Input: part model. Units: mm. Frame: model coordinates. A direction names the side the tool comes from. Coordinates: 2 decimals unless noted, no trailing zeros. Loops run counter-clockwise (first coordinate to the right, second up) from the corner with the lowest first, then second, coordinate; pieces in that order, holes last.
(1) Mould query, pull axis Y, two halves, no side actions, for faces 4 (the face through (-5.6, 9.4, -6)), 5 (the face through (2, 9, 3.175)), 6 (the face through (3, 9, 0)). Classes: released by +Y, released by -Y, zero draft, split by the parting line, or undercut.
(2) Section B-B, the plane x = 5. Return loops of the section in (y, z) (3 decimals), then the cut area to 3 significant figures.
(3) Contact query for flat-ended pins moving along their axis: P1, Ø5, axis at x = -4, z = -1.5, coming from the -Y side; P2, Ø0.6, axis at x = 3.5, y = 8.5, coming from the +Z side; P3, Ø3, axis at x = -3, y = 9, coming from the +Z side; P4, Ø3.5, axis at y = 5.7, z = -6.05, coming from the +X side. Output: stop coordinate, or through.
(4) Section A-A, the plane z = -6.05. Return loops of the section in (x, y), then the cut area to 3 significant figures.
(5) Set-up query: faces 1 (the face through (3.1, 9.5, 1.6)), 2 (the face through (3, 3, 0)), 3 (the face through (6.35, 8, -5)). Return all of +Z, -Z, +X, -X, +Y, -Y with unobstructed straight access to the full face (end or side cutting, diameter ignored); none if empty.
(6) Line query: L1, parallel to Y at x = 2.75, z = -6.05; L2, parallel to X at y = 9.5, z = -5; L3, parallel to Z at x = 1, y = 5.75 (3 decimals). Output: solid intervals per line, ascending.
(7) Section C-C, the plane y = 7.25. Return loops of the section in (x, z) (3 decimals), then the cut area to 3 significant figures.
Autodesk Inventor part; units mm, degrees
ref_plane "YZ Plane" through (0, 0, 0) normal (1, 0, 0) x (0, 1, 0)
ref_plane "XZ Plane" through (0, 0, 0) normal (0, 1, 0) x (-1, 0, 0)
ref_plane "XY Plane" through (0, 0, 0) normal (0, 0, 1) x (1, 0, 0)
sketch "Sketch1" plane through (0, 0, 0) normal (1, 0, 0) x (0, 1, 0)
  line L0 (0, 0) -> (11.4, 0)
  line L1 (11.4, 0) -> (11.4, -12.1)
  line L2 (11.4, -12.1) -> (0, -12.1)
  line L3 (0, -12.1) -> (0, 0)
  arc A0 (11.4, -2.9512) -> (11.4, -9.1488) centre (12.8006, -6.05) ccw
  point P0 (3.5, -5)
  dimension "d0" = 11.4
  dimension "d1" = 12.1
  dimension "d2" = 6.1976
  dimension "d3" = 2.9512
  dimension "d29" = 2
extrude "Extrusion1" add sketch "Sketch1" along normal blind 6.35
extrude "Extrusion2" add sketch "Sketch1" against normal blind 11.43 contours L1 A0
sketch "Sketch3" plane through (0, 0, 0) normal (-1, 0, 0) x (0, 0, 1)
  line L0 (0, 11.4) -> (0, 0)
  line L1 (0, 0) -> (-12.1, 0)
  point P0 (-6.05, 5.7)
  dimension "d19" = 12.1
  dimension "d20" = 6.05
  dimension "d30" = 11.4
  dimension "d31" = 5.7
sketch "Sketch6" plane through (0, 0, 0) normal (0, 0, 1) x (1, 0, 0)
  line L0 (6.35, 5.7) -> (0, 5.7)
  line L1 (0, 0) -> (0, 11.4)
  line L2 (6.35, 11.4) -> (6.35, 0)
  line L3 (0, 0) -> (6.35, 0)
  line L4 (0, 11.4) -> (6.35, 11.4)
  dimension "d33" = 11.4
  dimension "d46" = 5.7
hole "Hole2" at (0, 5.7, -6.05) direction (1, 0, 0) diameter 4 end through all
extrude "Extrusion8" add sketch "Sketch6" along normal blind 3.175 contours L0 L1 L4 L2
sketch "Sketch7" plane through (0, 0, 3.175) normal (0, 0, 1) x (1, 0, 0)
  line L0 (6.35, 11.4) -> (0, 11.4)
  line L1 (6.35, 5.7) -> (6.35, 11.4)
  point P0 (0, 0)
  point P1 (3.175, 8.55)
  dimension "d50" = 6.35
  dimension "d51" = 5.7
  dimension "d52" = 2.85
  dimension "d53" = 3.175
sketch "Sketch8" plane through (0, 0, 3.175) normal (0, 0, 1) x (1, 0, 0)
  circle A0 centre (3.175, 8.55) radius 0.9525
  line L0 (6.35, 11.4) -> (0, 11.4)
  line L1 (6.35, 5.7) -> (6.35, 11.4)
  point P0 (0, 0)
  dimension "d63" = 2.85
  dimension "d64" = 3.175
  dimension "d65" = 1.905
extrude "Extrusion9" cut sketch "Sketch8" against normal up to surface (3.175 mm away)
equation "\"d3\" = -0.5 * d2 + 0.5 * d1"
equation "\"d46\" = 0.5 * d33"
equation "\"d63\" = d52"
equation "\"d64\" = d53"
properties part number "end peice for slides"
Report:
1. face 4: released by -Y
1. face 5: zero draft
1. face 6: undercut
2. outline: (0, -12.1) - (11.4, -12.1) - (11.4, 3.175) - (5.7, 3.175) - (5.7, 0) - (0, 0) - close; hole circle Ø4 at (5.7, -6.05)
2. area: 143 mm2
3. P1: stops at y = 10.09
3. P2: stops at z = 0
3. P3: stops at z = -3.55
3. P4: passes through
4. outline: (-11.43, 9.4) - (0, 9.4) - (0, 7.7) - (6.35, 7.7) - (6.35, 11.4) - (-11.43, 11.4) - close; (0, 0) - (6.35, 0) - (6.35, 3.7) - (0, 3.7) - close
4. area: 69.9 mm2
5. face 1: +Z
5. face 2: +Z, +X, -X, -Y
5. face 3: +Z, -Z, +X, +Y, -Y
6. L1: y = 0 to 3.7, 7.7 to 11.4
6. L2: x = 0 to 6.35
6. L3: z = -12.1 to -8.049, -4.051 to 3.175
7. outline: (0, -12.1) - (6.35, -12.1) - (6.35, -7.314) - (0, -7.314) - close; (0, -4.786) - (6.35, -4.786) - (6.35, 3.175) - (0, 3.175) - close
7. area: 80.9 mm2
